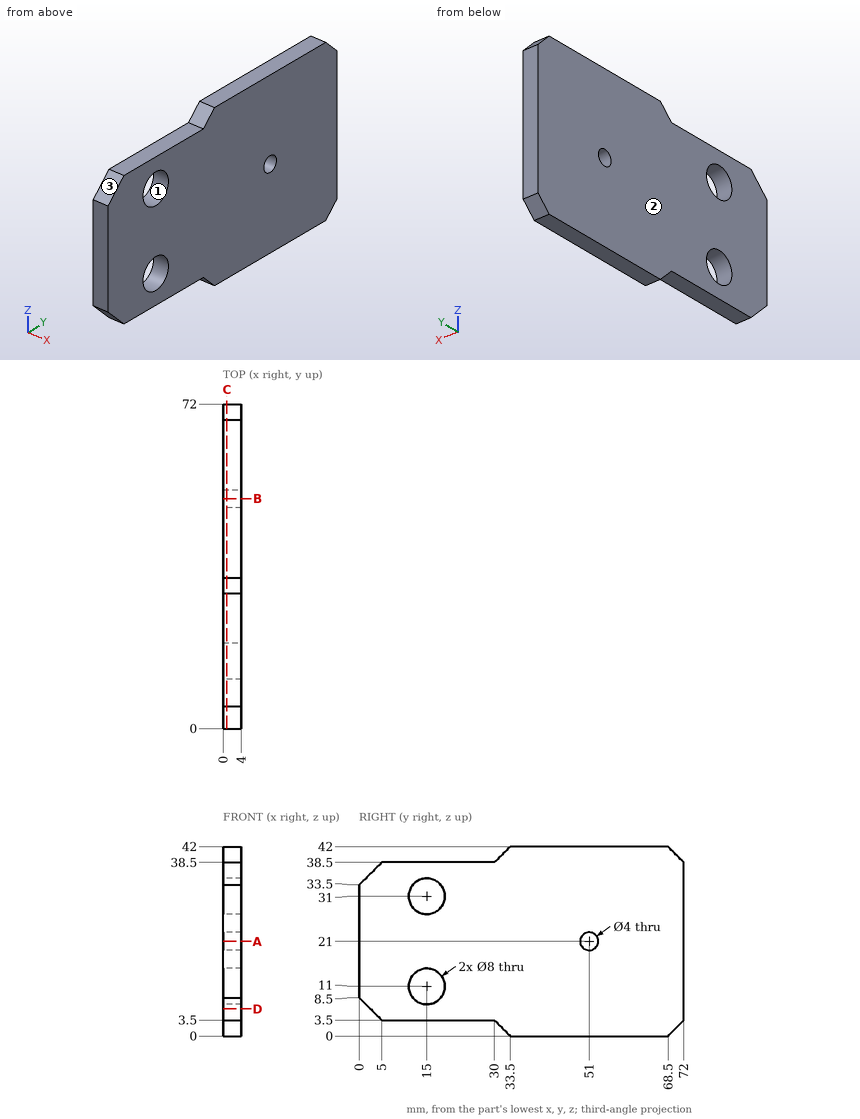
Design review of the part shown in the three views and the two pictorial views. Dimensions are in mm from the part's minimum x, y and z. Give positions to 0.01 mm unless a question says otherwise; leave off trailing zeros. Loops run counter-clockwise (first coordinate to the right, second up) from the corner with the lowest first, then second, coordinate; pieces in that order, holes last. Notation, with made-up numbers: (45, 73.25) -> (72, 73.25) arc R24 ccw to (72, 97.25) -> close; hole circle Ø4 at (2, -17). An arc over 180 degrees is marked (long way). Write each question's results on one line, items separated by ' | '.
1) Draft analysis for pull direction Z (two halves, no side actions). For the marked faces 1, 2 and 3, state which applies: pulls with the +Z half, pulls with the -Z half, needs draft (parallel to the pull), parting line crosses it, or undercut.
Conclusion:
face 1: undercut | face 2: needs draft | face 3: pulls with the +Z half
2) Take a section at A-A, the plane z = 21. Give the boundary of the cut face in (x, y).
Conclusion:
outline: (0, 0) -> (4, 0) -> (4, 49) -> (0, 49) -> close; (0, 53) -> (4, 53) -> (4, 72) -> (0, 72) -> close
3) Take a section at B-B, the plane y = 51. Give the boundary of the cut face in (x, z).
Conclusion:
outline: (0, 0) -> (4, 0) -> (4, 19) -> (0, 19) -> close; (0, 23) -> (4, 23) -> (4, 42) -> (0, 42) -> close
4) Take a section at D-D, the plane z = 6. Give the boundary of the cut face in (x, y).
Conclusion:
outline: (0, 2.5) -> (4, 2.5) -> (4, 72) -> (0, 72) -> close
5) Take a section at C-C, the plane x = 0.8. Give the boundary of the cut face in (y, z).
Conclusion:
outline: (0, 8.5) -> (5, 3.5) -> (30, 3.5) -> (33.5, 0) -> (68.5, 0) -> (72, 3.5) -> (72, 38.5) -> (68.5, 42) -> (33.5, 42) -> (30, 38.5) -> (5, 38.5) -> (0, 33.5) -> close; hole circle Ø8 at (15, 11); hole circle Ø8 at (15, 31); hole circle Ø4 at (51, 21)
6) Insertion check: pin 1 Ø5 at (y, z) = (15, 11) entering from -X; pin 2 Ø2 at (x, y) = (2, 15) entering from +Z; pin 3 Ø2 at (x, y) = (2, 22) entering from -Z. Each pin has a flat end and moves straight along its axis. Give the tip position at first contact, or say it passes through.
Conclusion:
pin 1: passes through | pin 2: stops at z = 38.5 | pin 3: stops at z = 3.5
7) For line 1 along Z through (x, y) = (2.85, 15); line 2 along Z through (x, y) = (1.1, 51); line 3 along Y through (x, z) = (1.65, 9.5), list the stretches that pass through material, from the lowest coordinate up. Write a range as from..to.
Conclusion:
line 1: z = 3.5..7, 15..27, 35..38.5 | line 2: z = 0..19, 23..42 | line 3: y = 0..11.29, 18.71..72
